```python
from build123d import *

# Parameters (mm, degrees)
SKETCH1_W              = 12.7
SKETCH1_H              = 234.95
BOSS_EXTRUDE1_DEPTH    = 3.175
SKETCH2_W              = 4.953
SKETCH2_H              = 12.319
CUT_EXTRUDE1_DEPTH     = 241.400131292
FILLET1_R              = 2.54
LPATTERN3_COUNT        = 9
LPATTERN3_PITCH        = 24.13
FILLET1_OF_LPATTERN3_R = 2.54
M4X0_7_TAPPED_HOLE1_D  = 3.3
BOSS_EXTRUDE2_START    = -3.175
SKETCH5_W              = 12.7
SKETCH5_H              = 6.35
BOSS_EXTRUDE2_DEPTH    = 6.35
M3X0_5_TAPPED_HOLE1_D  = 2.5
FILLET2_R              = 3.302
SKETCH8_R              = 2.5527
CUT_EXTRUDE2_DEPTH     = 241.463022105


with BuildPart() as part:
    # Sketch1 → Boss-Extrude1 (new, symmetric)
    with BuildSketch(Plane.XY):
        with Locations((-44.45, 117.475)):
            Rectangle(SKETCH1_W, SKETCH1_H)
    extrude(amount=BOSS_EXTRUDE1_DEPTH, both=True)

    # Sketch2 → Cut-Extrude1 (cut, symmetric)
    with BuildSketch(Plane.XY):
        with Locations((-48.3235, 19.91868)):
            Rectangle(SKETCH2_W, SKETCH2_H)
    cut_extrude1 = extrude(amount=CUT_EXTRUDE1_DEPTH, both=True, mode=Mode.SUBTRACT)

    # Fillet1
    fillet1_edges = [part.edges().sort_by_distance(p)[0] for p in [
        (-45.847, 26.07818, 0),
        (-45.847, 13.75918, 0),
    ]]
    fillet(fillet1_edges, radius=FILLET1_R)

    # LPattern3: Cut-Extrude1 ×9
    with Locations(*[(0, i * LPATTERN3_PITCH, 0) for i in range(1, LPATTERN3_COUNT)]):
        add(cut_extrude1, mode=Mode.SUBTRACT)

    # Fillet1 of LPattern3
    fillet1_of_lpattern3_edges = [part.edges().sort_by_distance(p)[0] for p in [
        (-45.847, 50.20818, 0),
        (-45.847, 37.88918, 0),
        (-45.847, 74.33818, 0),
        (-45.847, 62.01918, 0),
        (-45.847, 98.46818, 0),
        (-45.847, 86.14918, 0),
        (-45.847, 122.59818, 0),
        (-45.847, 110.27918, 0),
        (-45.847, 146.72818, 0),
        (-45.847, 134.40918, 0),
        (-45.847, 170.85818, 0),
        (-45.847, 158.53918, 0),
        (-45.847, 194.98818, 0),
        (-45.847, 182.66918, 0),
        (-45.847, 219.11818, 0),
        (-45.847, 206.79918, 0),
    ]]
    fillet(fillet1_of_lpattern3_edges, radius=FILLET1_OF_LPATTERN3_R)

    # M4x0.7 Tapped Hole1 (through all)
    with Locations(Plane.ZY.offset(50.8)):
        with Locations((0, 80.24368), (0, 176.76368)):
            Hole(M4X0_7_TAPPED_HOLE1_D / 2)

    # Sketch5 → Boss-Extrude2 (add)
    with BuildSketch(Plane.XY.offset(BOSS_EXTRUDE2_START)):
        with Locations((-31.75, 3.175)):
            Rectangle(SKETCH5_W, SKETCH5_H)
    extrude(amount=BOSS_EXTRUDE2_DEPTH)

    # M3x0.5 Tapped Hole1 (through all)
    with Locations(Plane.XY.offset(3.175)):
        with Locations((-41.275, 11.43), (-41.275, 158.75)):
            Hole(M3X0_5_TAPPED_HOLE1_D / 2)

    # Fillet2
    fillet2_edges = [part.edges().sort_by_distance(p)[0] for p in [
        (-38.1, 6.35, 0),
    ]]
    fillet(fillet2_edges, radius=FILLET2_R)

    # Sketch8 → Cut-Extrude2 (cut, through all)
    with BuildSketch(Plane.XY.offset(3.175)):
        with Locations((-42.926, 200.89368)):
            Circle(SKETCH8_R)
        with Locations((-42.926, 56.11368)):
            Circle(SKETCH8_R)
        with Locations((-42.926, 128.50368)):
            Circle(SKETCH8_R)
    extrude(amount=-CUT_EXTRUDE2_DEPTH, mode=Mode.SUBTRACT)


solid = part.part
```
Part model, mm, in its own coordinate system. A direction names the side the tool comes from. Give positions to 0.01 mm unless a question says otherwise; leave off trailing zeros. Write each loop counter-clockwise with the first axis right and the second up, starting at its lowest first coordinate (ties: lowest second). Pieces come first, ordered by that corner, then holes. Notation, with made-up numbers: (-4.75, 71) -> (27.25, 71) arc R15 ccw to (27.25, 95) -> close; hole circle Ø4 at (-27, -32). An arc over 180 degrees is marked (long way). Put each result on its own line as item: value. Start each with the question number.
Item 1: Cut at B-B (x = -28.25). List the corners of the cut face in (y, z) (3 decimals).
Item 2: Cut at C-C (y = 29). List the corners of the cut face in (x, z) (3 decimals).
Item 3: Pull direction Y, two halves, no side cores. Call faces 1 (the face through (-50.8, 153, 0)), 2 (the face through (-30, 6.35, 0)), 3 (the face through (-45.847, 213, 0)): pulls with the +Y half, pulls with the -Y half, needs draft (parallel to the pull), parting line crosses it, or undercut.
Item 4: Wall check: L1, parallel to Y at x = -38.25, z = -0.25; L2, parallel to Y at x = -44.25, z = 0; L3, parallel to Y at x = -43.75, z = -0.75. Give the ranges that are in metal, low to high. Write a range as [from, to].
Item 5: Cut at A-A (z = 0). State how many separate pieces and enclosed holes the cut face has, then the cut area to 3 significant figures.
Item 6: Which spindle directions (+Z, -Z, +X, -X, +Y, -Y) get a long thin tool onto all of the face, cutting with end or side? Do faces 4 (the face through (-45.476, 128.616, 0.044)), 5 (the face through (-45.847, 92, 0)). Say none if no direction does.
Item 7: Pin check, flat tips, straight feed: pin 1 Ø3 at (y, z) = (213, 1) entering from -X; pin 2 Ø3 at (y, z) = (80.24, 0) entering from -X; pin 3 Ø1 at (y, z) = (136, -1.5) entering from +X. Stop position of each tip, or through.
Answer list:
1. outline: (0, -3.175) -> (6.35, -3.175) -> (6.35, 3.175) -> (0, 3.175) -> close
2. outline: (-50.8, -3.175) -> (-38.1, -3.175) -> (-38.1, 3.175) -> (-50.8, 3.175) -> close
3. face 1: needs draft
3. face 2: pulls with the +Y half
3. face 3: undercut
4. L1: y = [0, 78.61], [81.87, 175.13], [178.39, 234.95]
4. L2: y = [0, 53.93], [58.3, 78.59], [81.89, 126.32], [130.69, 175.11], [178.41, 198.71], [203.08, 234.95]
4. L3: y = [0, 53.7], [58.53, 78.77], [81.71, 126.09], [130.92, 175.29], [178.23, 198.48], [203.31, 234.95]
5. separate pieces: 3
5. enclosed holes: 5
5. area: 2,390 mm2
6. face 4: +Z, -Z
6. face 5: +Z, -Z, -X
7. pin 1: stops at x = -45.85
7. pin 2: passes through
7. pin 3: stops at x = -38.1
